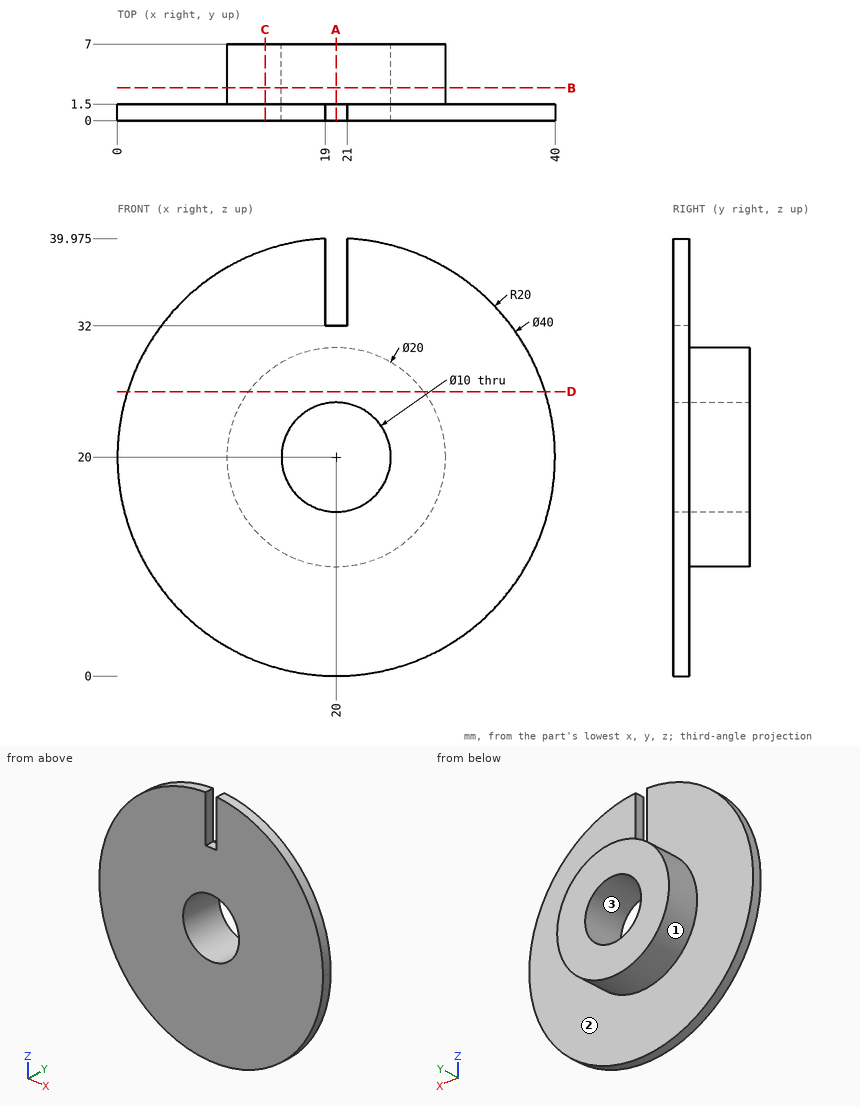
The drawing under review shows one solid part. Ordinate dimensions are in mm from its lowest x, y, z. Give positions to 0.01 mm unless a question says otherwise; leave off trailing zeros. Write each loop counter-clockwise with the first axis right and the second up, starting at its lowest first coordinate (ties: lowest second). Pieces come first, ordered by that corner, then holes. Notation, with made-up numbers: (-37, 51) -> (22, 51) arc R27 ccw to (22, 89) -> close; hole circle Ø5 at (18, 62). An arc over 180 degrees is marked (long way). Put each result on its own line as item: value.
(1) The part is to be moulded in two halves that separate along X. For the marked faces 1, 2 and 3, say which applies: pulls with the +X half, pulls with the -X half, needs draft (parallel to the pull), parting line crosses it, or undercut.
Results are:
face 1: parting line crosses it
face 2: needs draft
face 3: undercut
(2) To check wall thickness, follow probe 1 along Z at (x, y) = (20, 1.75); probe 2 along Y at (x, z) = (31, 27.5); probe 3 along Z at (x, y) = (23.5, 1.25). State the ranges of each line that lie inside material, in increasing order. Write a range as from..to.
Results are:
probe 1: 10..15, 25..30
probe 2: 0..1.5
probe 3: 0.31..16.43, 23.57..39.69
(3) We need section A-A, the plane x = 20. Give the boundary of the cut face in (y, z).
Results are:
outline: (0, 0) -> (1.5, 0) -> (1.5, 10) -> (7, 10) -> (7, 15) -> (0, 15) -> close; (0, 25) -> (7, 25) -> (7, 30) -> (1.5, 30) -> (1.5, 32) -> (0, 32) -> close
(4) We need section C-C, the plane x = 13.5. Give the boundary of the cut face in (y, z), and give its area (3 significant figures).
Results are:
outline: (0, 1.09) -> (1.5, 1.09) -> (1.5, 12.4) -> (7, 12.4) -> (7, 27.6) -> (1.5, 27.6) -> (1.5, 38.91) -> (0, 38.91) -> close
area: 140 mm²
(5) We need section D-D, the plane z = 26. Give the boundary of the cut face in (x, y), and give its area (3 significant figures).
Results are:
outline: (0.92, 0) -> (39.08, 0) -> (39.08, 1.5) -> (28, 1.5) -> (28, 7) -> (12, 7) -> (12, 1.5) -> (0.92, 1.5) -> close
area: 145 mm²
(6) We need section B-B, the plane y = 3. Give the boundary of the cut face in (x, z), and give its area (3 significant figures).
Results are:
outline: circle Ø20 at (20, 20); hole circle Ø10 at (20, 20)
area: 236 mm²
(7) For pin 1 Ø3 at (x, z) = (7, 20) entering from +Y; pin 2 Ø0.8 at (x, y) = (20.5, 1) entering from +Z; pin 3 Ø3 at (x, y) = (21.5, 1) entering from -Z, all flat-tipped, find the tip position at first contact; note any pin that passes through.
Results are:
pin 1: y = 1.5
pin 2: z = 32
pin 3: z = 0
